from build123d import *

# Parameters (mm, degrees)
F0_W      = 525
F0_H      = 525
F0_W_2    = 387
F0_H_2    = 387
F1_DEPTH  = 7
F2_DEPTH  = 30
F4_DEPTH  = 7
F7_DEPTH  = 25
F8_D      = 5
F9_D      = 5
F10_D     = 5
F11_D     = 5
F12_D     = 5
F13_R     = 2.5
F13_R_2   = 7.5
F14_DEPTH = 10


# Not quite as in the source:
# - a feature names something its author has since deleted; it is built from what else it names


with BuildPart() as f1:
    # F0 (on Top) → F1 (new body)
    with BuildSketch(Plane.XY):
        Rectangle(F0_W, F0_H)
        Rectangle(F0_W_2, F0_H_2, mode=Mode.SUBTRACT)
    extrude(amount=F1_DEPTH)

    # F0 (on Top) → F2 (join)
    with BuildSketch(Plane.XY):
        Rectangle(F0_W_2, F0_H_2)
        Polygon((-187.5, -6.596e-07), (-187.5, 187.5), (-6.149e-07, 187.5), (187.5, 187.5), (187.5, 0), (187.5, -187.5), (-6.893e-07, -187.5), (-187.5, -187.5), align=None, mode=Mode.SUBTRACT)
    extrude(amount=F2_DEPTH)

    # F3 (on face) → F4 (join)
    with BuildSketch(Plane.XY.offset(30)):
        with BuildLine():
            ThreePointArc((-187.5, 47.8121323515), (-136.8251621596, 136.8251621596), (-47.8121323515, 187.5))
            Line((-47.8121323515, 187.5), (-187.5, 187.5))
            Line((-187.5, 187.5), (-187.5, 47.8121323515))
        make_face()
        with BuildLine():
            ThreePointArc((-6.149e-07, 187.5), (132.5825212551, 132.5825216899), (187.5, 0))
            Line((187.5, 0), (187.5, 47.8121323515))
            ThreePointArc((187.5, 47.8121323515), (136.8251621596, 136.8251621596), (47.8121323515, 187.5))
            Line((47.8121323515, 187.5), (-6.149e-07, 187.5))
        make_face()
        with BuildLine():
            ThreePointArc((-187.5, -6.596e-07), (-132.5825219231, 132.5825210219), (-6.149e-07, 187.5))
            Line((-6.149e-07, 187.5), (-47.8121323515, 187.5))
            ThreePointArc((-47.8121323515, 187.5), (-136.8251621596, 136.8251621596), (-187.5, 47.8121323515))
            Line((-187.5, 47.8121323515), (-187.5, -6.596e-07))
        make_face()
        with BuildLine():
            Line((-47.8121323515, -187.5), (-6.893e-07, -187.5))
            ThreePointArc((-6.893e-07, -187.5), (-132.582521483, -132.582521462), (-187.5, -6.596e-07))
            Line((-187.5, -6.596e-07), (-187.5, -47.8121323515))
            ThreePointArc((-187.5, -47.8121323515), (-136.8251621596, -136.8251621596), (-47.8121323515, -187.5))
        make_face()
        with BuildLine():
            Line((187.5, -47.8121323515), (187.5, 0))
            ThreePointArc((187.5, 0), (132.5825212288, -132.5825217162), (-6.893e-07, -187.5))
            Line((-6.893e-07, -187.5), (47.8121323515, -187.5))
            ThreePointArc((47.8121323515, -187.5), (136.8251621596, -136.8251621596), (187.5, -47.8121323515))
        make_face()
        with BuildLine():
            ThreePointArc((47.8121323515, 187.5), (136.8251621596, 136.8251621596), (187.5, 47.8121323515))
            Line((187.5, 47.8121323515), (187.5, 187.5))
            Line((187.5, 187.5), (47.8121323515, 187.5))
        make_face()
        with BuildLine():
            Line((187.5, -187.5), (187.5, -47.8121323515))
            ThreePointArc((187.5, -47.8121323515), (136.8251621596, -136.8251621596), (47.8121323515, -187.5))
            Line((47.8121323515, -187.5), (187.5, -187.5))
        make_face()
        with BuildLine():
            Line((-187.5, -187.5), (-47.8121323515, -187.5))
            ThreePointArc((-47.8121323515, -187.5), (-136.8251621596, -136.8251621596), (-187.5, -47.8121323515))
            Line((-187.5, -47.8121323515), (-187.5, -187.5))
        make_face()
    extrude(amount=-F4_DEPTH)

    # F5 (on Front) → F6 (revolve)
    with BuildSketch(Plane.XZ):
        Polygon((-109.5, 240), (-193.5, 30), (-149.8333333333, 30), (-91.5, 240), align=None)
    revolve(axis=Axis((0, 0, 120), (0, 0, 1)))

    # F7 (add): a face of the model
    f7_faces = [f1.faces().sort_by_distance(p)[0] for p in [
        (94.5971277016, 0, 240),
    ]]
    extrude(f7_faces, amount=F7_DEPTH)

    # F8 (through all)
    with Locations(Plane(origin=(0, 0, 0), x_dir=(1, 0, 0), z_dir=(0, 0, -1))):
        with Locations((-157.5, -157.5)):
            Hole(F8_D / 2)

    # F9 (through all)
    with Locations(Plane(origin=(0, 0, 0), x_dir=(1, 0, 0), z_dir=(0, 0, -1))):
        with Locations((157.5, -157.5)):
            Hole(F9_D / 2)

    # F10 (through all)
    with Locations(Plane(origin=(0, 0, 0), x_dir=(1, 0, 0), z_dir=(0, 0, -1))):
        with Locations((-157.5, 157.5)):
            Hole(F10_D / 2)

    # F11 (through all)
    with Locations(Plane(origin=(0, 0, 0), x_dir=(1, 0, 0), z_dir=(0, 0, -1))):
        with Locations((157.5, 157.5)):
            Hole(F11_D / 2)

    # F12 (through all)
    with Locations(Plane(origin=(0, 0, 0), x_dir=(1, 0, 0), z_dir=(0, 0, -1))):
        with Locations((-203, -203), (0, -203), (203, -203), (203, 0), (203, 203), (0, 203), (-203, 203), (-203, 0)):
            Hole(F12_D / 2)

    # F13 (on face) → F14 (cut)
    with BuildSketch(Plane.XY.offset(30)):
        with Locations((157.5, -157.5)):
            Circle(F13_R)
        with Locations((-157.5, -157.5)):
            Circle(F13_R_2)
        with Locations((-157.5, 157.5)):
            Circle(F13_R_2)
        with Locations((157.5, 157.5)):
            Circle(F13_R_2)
    extrude(amount=F14_DEPTH, mode=Mode.SUBTRACT)


solid = f1.part
Can you work these out from the model? Positions are in its coordinate system, mm. A direction names the side the tool comes from. Give positions to 0.01 mm unless a question says otherwise; leave off trailing zeros. Loops run counter-clockwise (first coordinate to the right, second up) from the corner with the lowest first, then second, coordinate; pieces in that order, holes last. Notation, with made-up numbers: M 40,5.25 L 89,5.25 A14 ccw 89,25.25 Z; hole C -33,58 d11. An arc over 180 degrees is marked long. One line per item, written item: value. Start each with the question number.
1) Thinking about a two-plate mould opening in Y: for faces 5 (the face through (-127.26, -40.076, 180.197)), 6 (the face through (-3, 187.5, 11)), 7 (the face through (-3, -193.5, 18)), which applies, +Y half, -Y half, draft (parallel to the pull), parting line (faces both ways), or undercut?
2) On a 3-axis mill with a long thin cutter (end or side, diameter ignored), from which of +Z, -Z, +X, -X, +Y, -Y can I reach the whole of each face in a straight line? I mean faces 1 (the face through (146, 155, 30)), 2 (the face through (3, -187.5, 11)), 3 (the face through (-3, 193.5, 18)), 4 (the face through (-155, -146, 30)). Say none if no direction works.
3) If we section it at B-B, the plane z = 67: Write out the boundary of the cut face in (x, y), and give its area (3 significant figures).
4) I'm going to push flat-ended pins straight in: pin 1 (11.5 mm diameter, centred on y = -81.5, z = 13, fed in from -X); pin 2 (4.5 mm diameter, centred on x = -203, y = -203, fed in from -Z); pin 3 (8 mm diameter, centred on x = -79, z = 201.5, fed in from -Y); pin 4 (12 mm diameter, centred on y = -101, z = 211.5, fed in from -X). Where does each tip first touch, or does it pass through?
5) If we section it at A-A, the plane z = 130: Write out the boundary of the cut face in (x, y).
6) If I drill on line 1 (X direction, y = 203, z = 1.5); line 2 (Y direction, x = 0, z = 259), over which ranges is the centre line in solid material (lowest first)? Write a range as [from, to].
Completed:
1. face 5: parting line
1. face 6: undercut
1. face 7: -Y half
2. face 1: +Z, +X, +Y
2. face 2: -Z
2. face 3: +Z, +X, -X, +Y
2. face 4: +Z, -X, -Y
3. outline: C 0,0 d357.4; hole C 0,0 d279.11
3. area: 39,100 mm^2
4. pin 1: stops at x = -193.5
4. pin 2: passes through
4. pin 3: stops at y = -100.48
4. pin 4: stops at x = -75.71
5. outline: C 0,0 d307; hole C 0,0 d244.11
6. line 1: x = [-262.5, -205.5], [-200.5, -2.5], [2.5, 200.5], [205.5, 262.5]
6. line 2: y = [-109.5, -91.5], [91.5, 109.5]
